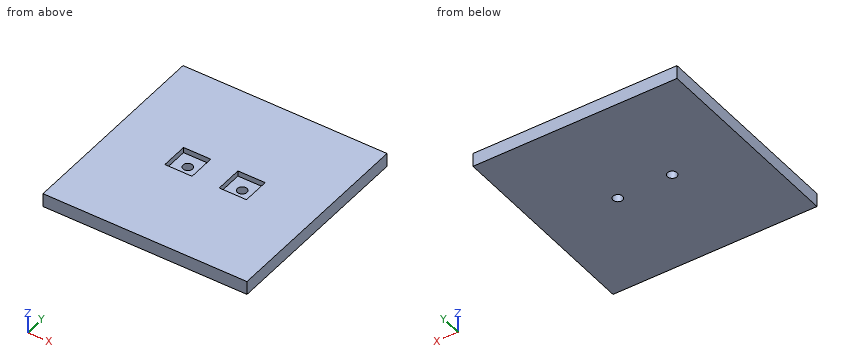
from build123d import *

# Parameters (mm, degrees)
SKETCH_1_W      = 75
SKETCH_1_H      = 75
SKETCH_1_W_2    = 10
SKETCH_1_H_2    = 10
EXTRUDE_1_DEPTH = 5
SKETCH_1_8_W    = 10
SKETCH_1_8_H    = 10
SKETCH_1_8_R    = 1.75
EXTRUDE_2_DEPTH = 3


with BuildPart() as part:
    # Sketch 1 → Extrude 1 (new body)
    # profile 1 of 2: a face of its own
    with BuildSketch(Plane.XY):
        Rectangle(SKETCH_1_W, SKETCH_1_H)
        Polygon((-15, 5), (-15, -5), (-5, -5), (5, -5), (15, -5), (15, 5), (5, 5), (-5, 5), align=None, mode=Mode.SUBTRACT)
    # profile 2 of 2: a face of its own
    with BuildSketch(Plane.XY):
        Rectangle(SKETCH_1_W_2, SKETCH_1_H_2)
    extrude(amount=EXTRUDE_1_DEPTH)

    # Sketch 1_8 → Extrude 2 (add)
    # profile 1 of 2: a face of its own
    with BuildSketch(Plane.XY):
        with Locations((-10, 0)):
            Rectangle(SKETCH_1_8_W, SKETCH_1_8_H)
        with Locations((-10, 0)):
            Circle(SKETCH_1_8_R, mode=Mode.SUBTRACT)
    # profile 2 of 2: a face of its own
    with BuildSketch(Plane.XY):
        with Locations((10, 0)):
            Rectangle(SKETCH_1_8_W, SKETCH_1_8_H)
        with Locations((10, 0)):
            Circle(SKETCH_1_8_R, mode=Mode.SUBTRACT)
    extrude(amount=EXTRUDE_2_DEPTH)


solid = part.part
For this review, take the finished solid that the model builds, in its own axes (mm). Round coordinates to 2 decimals unless told otherwise and drop trailing zeros. Order: outer loops, then holes, each group sorted by start corner. A loop starts at its lowest first (then second) coordinate and runs counter-clockwise, first axis right, second up. Notation, with made-up numbers: M -7,69.25 L 20,69.25 A18 cw 20,87.25 Z; hole C 15.25,-12 d4. An arc over 180 degrees is marked long. Use a Markdown table: item, result. Add a question column.
Item 1: Add section A-A, the plane y = 0. Give the boundary of the cut face in (x, z), then the cut area to 3 significant figures.
Item 2: Add section C-C, the plane z = 3.8. Give the boundary of the cut face in (x, y), then the cut area to 4 significant figures.
Item 3: Insertion check: pin 1 (5 mm diameter, centred on x = -9, y = -0.5, fed in from +Z). The pin has a flat end and moves straight along its axis. Give the tip position at first contact, or say it passes through.
Item 4: Add section B-B, the plane x = -10. Give the boundary of the cut face in (y, z), then the cut area to 4 significant figures.
Item 5: To check wall thickness, follow line 1 along Y through (x, z) = (10, 1.7); line 2 along Z through (x, y) = (13, 2). State the ranges of each line that lie inside material, in increasing order.
Geometry results:
| question | item | result |
|---|---|---|
| 1 | outline | M -37.5,0 L -11.75,0 L -11.75,3 L -15,3 L -15,5 L -37.5,5 Z; M -8.25,0 L 8.25,0 L 8.25,3 L 5,3 L 5,5 L -5,5 L -5,3 L -8.25,3 Z; M 11.75,0 L 37.5,0 L 37.5,5 L 15,5 L 15,3 L 11.75,3 Z |
| 1 | area | 314 mm² |
| 2 | outline | M -37.5,-37.5 L 37.5,-37.5 L 37.5,37.5 L -37.5,37.5 Z; hole M -15,-5 L -5,-5 L -5,5 L -15,5 Z; hole M 5,-5 L 15,-5 L 15,5 L 5,5 Z |
| 2 | area | 5,425 mm² |
| 3 | pin 1 | stops at z = 3 |
| 4 | outline | M -37.5,0 L -1.75,0 L -1.75,3 L -5,3 L -5,5 L -37.5,5 Z; M 1.75,0 L 37.5,0 L 37.5,5 L 5,5 L 5,3 L 1.75,3 Z |
| 4 | area | 344.5 mm² |
| 5 | line 1 | y = -37.5 to -1.75, 1.75 to 37.5 |
| 5 | line 2 | z = 0 to 3 |
